from build123d import *

# Parameters (mm, degrees)
SKETCH_2_R               = 1.6
CUT_EXTRUDE_1_DEPTH      = 3
PATTERN_CIRCULAR_1_COUNT = 4
CHAMFER_1_SIZE           = 0.4


with BuildPart() as part:
    # Эскиз1 → Повернуть1 (revolve)
    with BuildSketch(Plane(origin=(0, 0, 0), x_dir=(1, 0, 0), z_dir=(0, 1, 0))):
        Polygon((-18, 0), (-18, 3), (-12.5, 3), (-12.5, 13), (-6, 13), (-6, 10), (-9.5, 10), (-9.5, 0), align=None)
    revolve(axis=Axis((0, 0, 0), (0, 0, -1)))

    # Эскиз2 → Вырез-Вытянуть1 (cut)
    with BuildSketch(Plane.XY):
        with Locations((10.606601718, 10.606601718)):
            Circle(SKETCH_2_R)
    cut_extrude_1 = extrude(amount=-CUT_EXTRUDE_1_DEPTH, mode=Mode.SUBTRACT)

    # Круговой массив1: Вырез-Вытянуть1 ×4 about axis
    pattern_circular_1_axis = Axis((0, 0, 0), (0, 0, 1))
    for i in range(1, PATTERN_CIRCULAR_1_COUNT):
        add(cut_extrude_1.rotate(pattern_circular_1_axis, i * 360 / PATTERN_CIRCULAR_1_COUNT), mode=Mode.SUBTRACT)

    # Фаска1
    chamfer_1_edges = [part.edges().sort_by_distance(p)[0] for p in [
        (9.5, 0, 0),
        (12.5, 0, -13),
    ]]
    chamfer(chamfer_1_edges, length=CHAMFER_1_SIZE)


solid = part.part
Read the model definition and answer for the solid it produces. Units are mm, in the model's axes. A direction names the side the tool comes from. Round coordinates to 2 decimals unless told otherwise and drop trailing zeros. Write each loop counter-clockwise with the first axis right and the second up, starting at its lowest first coordinate (ties: lowest second). Pieces come first, ordered by that corner, then holes. Notation, with made-up numbers: (-1, -24) - (30, -24) arc R17 ccw to (30, -9) - close; hole circle Ø9 at (-30, 1.5). An arc over 180 degrees is marked (long way). One line per question, with ' | ' between items. Start each with the question number.
1. Section A-A (y = 0) is taken. Determine the outline of the cut face in (x, z).
2. Find the intervals of material crossed by probe 1 along Y at (x, z) = (0, -7.25); probe 2 along Y at (x, z) = (-8.5, -4); probe 3 along Z at (x, y) = (1.5, 14.5), in increasing order. Write a range as [from, to].
3. For faces 5 (the face through (-11.345, -9.187, -1.479)), 6 (the face through (-4.38, -8.43, -5.13)), determine the directions among +Z, -Z, +X, -X, +Y, -Y from which every point of the face is accessible in a straight line to the end or side of a thin tool.
4. Section C-C (z = -6) is taken. Determine the outline of the cut face in (x, y).
5. Each of these flat-tipped pins is pushed along its axis until it touches: pin 1 (6 mm diameter, centred on x = -12.5, z = -4, fed in from -Y); pin 2 (3.5 mm diameter, centred on x = 10.61, y = -10.61, fed in from -Z); pin 3 (6 mm diameter, centred on x = 6.5, y = -11, fed in from -Z); pin 4 (4 mm diameter, centred on x = 2.5, z = -2, fed in from -Y). Where does it stop, or does it pass through?
6. For a pull along Y with two mould halves and no side action, classify faces 1 (the face through (6, 0, -11)), 2 (the face through (-11.923, 3.755, -7.867)), 3 (the face through (12.3, -3.7, -3)), 4 (the face through (-9.187, 11.345, -1.479)) as +Y half, -Y half, draft (parallel to the pull), parting line (faces both ways), or undercut.
Filled in:
1) outline: (-18, -3) - (-12.5, -3) - (-12.5, -12.6) - (-12.1, -13) - (-6, -13) - (-6, -10) - (-9.5, -10) - (-9.5, -0.4) - (-9.9, 0) - (-18, 0) - close; (6, -13) - (12.1, -13) - (12.5, -12.6) - (12.5, -3) - (18, -3) - (18, 0) - (9.9, 0) - (9.5, -0.4) - (9.5, -10) - (6, -10) - close
2) probe 1: [-12.5, -9.5], [9.5, 12.5] | probe 2: [-9.17, -4.24], [4.24, 9.17] | probe 3: [-3, 0]
3) face 5: +Z, -Z | face 6: +Z
4) outline: circle Ø25 at (0, 0); hole circle Ø19 at (0, 0)
5) pin 1: y = -15.18 | pin 2: z = -3 | pin 3: z = -13 | pin 4: y = -17.99
6) face 1: undercut | face 2: parting line | face 3: draft | face 4: undercut
